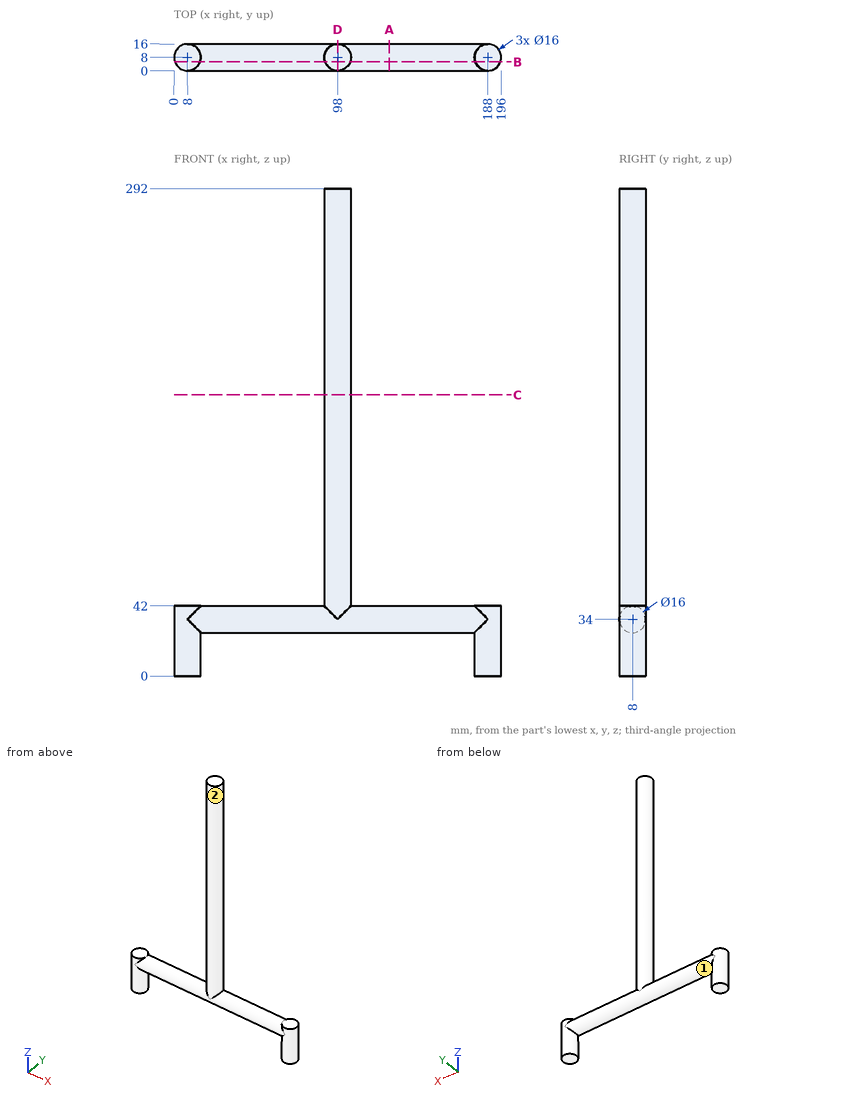
Input: dimensioned drawing with shaded views. Units: mm. Origin: part minimum x, y, z. A direction names the side the tool comes from. Round coordinates to 2 decimals unless told otherwise and drop trailing zeros. Order: outer loops, then holes, each group sorted by start corner. A loop starts at its lowest first (then second) coordinate and runs counter-clockwise, first axis right, second up.
Q1. Section A-A, the plane x = 129. Output: boundary loops of the cut face in (y, z), and give its area (3 significant figures).
Result sheet:
outline: circle Ø16 at (8, 34)
area: 201 mm2
Q2. Material intervals for probe 1 along X at (y, z) = (9, 172); probe 2 along X at (y, z) = (7.75, 240); probe 3 along Z at (x, y) = (144, 7.75), sorted ascending.
Result sheet:
probe 1: x = 90.06 to 105.94
probe 2: x = 90 to 106
probe 3: z = 26 to 42
Q3. Access query for the marked faces 1 and 2. Directions: +Z, -Z, +X, -X, +Y, -Y. A direction counts if a zero-diameter tool reaches every point of the face in a straight line with its end or side. Return the directions, or none.
Result sheet:
face 1: none
face 2: +Z
Q4. Pin query (flat end, axial travel): pin 1 (5 mm diameter, centred on y = 8, z = 182.5, fed in from -X); pin 2 (1 mm diameter, centred on y = 9, z = 135.5, fed in from +X); pin 3 (5 mm diameter, centred on x = 91, z = 258, fed in from +Y). Return the tip coordinate at first contact, or that it passes through.
Result sheet:
pin 1: stops at x = 90
pin 2: stops at x = 105.98
pin 3: stops at y = 14.61
Q5. Section C-C, the plane z = 168.5. Output: boundary loops of the cut face in (x, y).
Result sheet:
outline: circle Ø16 at (98, 8)
Q6. Section D-D, the plane x = 98. Output: boundary loops of the cut face in (y, z).
Result sheet:
outline: (0, 34) arc R8 ccw to (16, 34) - (16, 292) - (0, 292) - close
Q7. Section B-B, the plane y = 5.25. Output: boundary loops of the cut face in (x, z).
Result sheet:
outline: (0.49, 0) - (15.51, 0) - (15.51, 26.49) - (180.49, 26.49) - (180.49, 0) - (195.51, 0) - (195.51, 42) - (180.49, 42) - (180.49, 41.51) - (105.51, 41.51) - (105.51, 292) - (90.49, 292) - (90.49, 41.51) - (15.51, 41.51) - (15.51, 42) - (0.49, 42) - close
